from build123d import *

# Parameters (mm, degrees)
SKETCH1_W               = 20
SKETCH1_H               = 20
SKETCH1_R               = 1.5
SKETCH1_R_2             = 8
BOSS_EXTRUDE1_DEPTH     = 2.5
SKETCH2_R               = 3.175
BOSS_EXTRUDE2_DEPTH     = 20
CUT_EXTRUDE2_DEPTH      = 27.119915773
CUT_EXTRUDE2_DEPTH_BACK = 27.119915773
SKETCH1_3_R             = 1.5


with BuildPart() as part:
    # Sketch1 → Boss-Extrude1 (new body)
    # profile 1 of 18: a face of its own
    with BuildSketch(Plane(origin=(0, 0, 0), x_dir=(1, 0, 0), z_dir=(0, 1, 0))):
        with Locations((0, -10)):
            Rectangle(SKETCH1_W, SKETCH1_H)
        with Locations((0, -2)):
            Circle(SKETCH1_R, mode=Mode.SUBTRACT)
        with Locations((0, -10)):
            Circle(SKETCH1_R_2, mode=Mode.SUBTRACT)
        with Locations((8, -10)):
            Circle(SKETCH1_R, mode=Mode.SUBTRACT)
        with Locations((0, -18)):
            Circle(SKETCH1_R, mode=Mode.SUBTRACT)
        with Locations((-8, -10)):
            Circle(SKETCH1_R, mode=Mode.SUBTRACT)
    # profile 2 of 18: a face of its own
    with BuildSketch(Plane(origin=(0, 0, 0), x_dir=(1, 0, 0), z_dir=(0, 1, 0))):
        with Locations((8, -10)):
            Circle(SKETCH1_R)
    # profile 3 of 18: a face of its own
    with BuildSketch(Plane(origin=(0, 0, 0), x_dir=(1, 0, 0), z_dir=(0, 1, 0))):
        with Locations((0, -18)):
            Circle(SKETCH1_R)
    # profile 4 of 18: a face of its own
    with BuildSketch(Plane(origin=(0, 0, 0), x_dir=(1, 0, 0), z_dir=(0, 1, 0))):
        with Locations((-8, -10)):
            Circle(SKETCH1_R)
    # profile 5 of 18: a face of its own
    with BuildSketch(Plane(origin=(0, 0, 0), x_dir=(1, 0, 0), z_dir=(0, 1, 0))):
        with Locations((0, -10)):
            Circle(SKETCH1_R_2)
    # profile 6 of 18: a face of its own
    with BuildSketch(Plane(origin=(0, 0, 0), x_dir=(1, 0, 0), z_dir=(0, 1, 0))):
        with Locations((0, -2)):
            Circle(SKETCH1_R)
    # profile 7 of 18: a face of its own
    with BuildSketch(Plane(origin=(0, 0, 0), x_dir=(1, 0, 0), z_dir=(0, 1, 0))):
        with Locations((0, -10)):
            Circle(SKETCH1_R_2)
    # profile 8 of 18: a face of its own
    with BuildSketch(Plane(origin=(0, 0, 0), x_dir=(1, 0, 0), z_dir=(0, 1, 0))):
        with Locations((8, -10)):
            Circle(SKETCH1_R)
    # profile 9 of 18: a face of its own
    with BuildSketch(Plane(origin=(0, 0, 0), x_dir=(1, 0, 0), z_dir=(0, 1, 0))):
        with Locations((0, -10)):
            Circle(SKETCH1_R_2)
    # profile 10 of 18: a face of its own
    with BuildSketch(Plane(origin=(0, 0, 0), x_dir=(1, 0, 0), z_dir=(0, 1, 0))):
        with Locations((0, -18)):
            Circle(SKETCH1_R)
    # profile 11 of 18: a face of its own
    with BuildSketch(Plane(origin=(0, 0, 0), x_dir=(1, 0, 0), z_dir=(0, 1, 0))):
        with Locations((0, -10)):
            Circle(SKETCH1_R_2)
    # profile 12 of 18: a face of its own
    with BuildSketch(Plane(origin=(0, 0, 0), x_dir=(1, 0, 0), z_dir=(0, 1, 0))):
        with Locations((0, -18)):
            Circle(SKETCH1_R)
    # profile 13 of 18: a face of its own
    with BuildSketch(Plane(origin=(0, 0, 0), x_dir=(1, 0, 0), z_dir=(0, 1, 0))):
        with Locations((0, -10)):
            Circle(SKETCH1_R_2)
    # profile 14 of 18: a face of its own
    with BuildSketch(Plane(origin=(0, 0, 0), x_dir=(1, 0, 0), z_dir=(0, 1, 0))):
        with Locations((-8, -10)):
            Circle(SKETCH1_R)
    # profile 15 of 18: a face of its own
    with BuildSketch(Plane(origin=(0, 0, 0), x_dir=(1, 0, 0), z_dir=(0, 1, 0))):
        with Locations((0, -10)):
            Circle(SKETCH1_R_2)
    # profile 16 of 18: a face of its own
    with BuildSketch(Plane(origin=(0, 0, 0), x_dir=(1, 0, 0), z_dir=(0, 1, 0))):
        with Locations((-8, -10)):
            Circle(SKETCH1_R)
    # profile 17 of 18: a face of its own
    with BuildSketch(Plane(origin=(0, 0, 0), x_dir=(1, 0, 0), z_dir=(0, 1, 0))):
        with Locations((0, -10)):
            Circle(SKETCH1_R_2)
    # profile 18 of 18: a face of its own
    with BuildSketch(Plane(origin=(0, 0, 0), x_dir=(1, 0, 0), z_dir=(0, 1, 0))):
        with Locations((8, -10)):
            Circle(SKETCH1_R)
    extrude(amount=BOSS_EXTRUDE1_DEPTH)

    # Sketch2 → Boss-Extrude2 (add)
    with BuildSketch(Plane.ZY.offset(10)):
        with BuildLine():
            Line((0, 0), (20, 0))
            Line((20, 0), (20, -3.5))
            ThreePointArc((20, -3.5), (10, -13.5), (0, -3.5))
            Line((0, -3.5), (0, 0))
        make_face()
        with Locations((10, -3.5)):
            Circle(SKETCH2_R, mode=Mode.SUBTRACT)
    extrude(amount=-BOSS_EXTRUDE2_DEPTH)

    # Sketch1<3> → Cut-Extrude2 (cut, two sides: drawn at the far end of the back side and taken through both)
    with BuildSketch(Plane(origin=(0, 0, 0), x_dir=(1, 0, 0), z_dir=(0, 1, 0)).offset(-CUT_EXTRUDE2_DEPTH_BACK)):
        with Locations(Location((8, -10, 0), (0, 0, 270))):
            Circle(SKETCH1_3_R)
        with Locations(Location((0, -18, 0), (0, 0, 270))):
            Circle(SKETCH1_3_R)
        with Locations(Location((-8, -10, 0), (0, 0, 270))):
            Circle(SKETCH1_3_R)
        with Locations(Location((0, -2, 0), (0, 0, 270))):
            Circle(SKETCH1_3_R)
    extrude(amount=CUT_EXTRUDE2_DEPTH + CUT_EXTRUDE2_DEPTH_BACK, mode=Mode.SUBTRACT)


solid = part.part
Design review of the part built by this model. Coordinates are the model's own, in mm. Coordinates: 2 decimals unless noted, no trailing zeros. Loops run counter-clockwise (first coordinate to the right, second up) from the corner with the lowest first, then second, coordinate; pieces in that order, holes last.
Item 1: Draft analysis for pull direction Z (two halves, no side actions). For faces 1 (the flat face through (10, -7, 10)), 2 (the cylindrical face through (6.536, 0.877, 9.675)), 3 (the flat face through (0, 0, 20)), state which applies: pulls with the +Z half, pulls with the -Z half, needs draft (parallel to the pull), parting line crosses it, or undercut.
Completed:
face 1: needs draft
face 2: undercut
face 3: pulls with the +Z half
Item 2: Add section A-A (z = 2). Write out the cut boundary in (x, y), and give its area (3 significant figures).
Completed:
outline: (-10, -9.5) - (-1.5, -9.5) - (-1.5, 2.5) - (-10, 2.5) - close; (1.5, -9.5) - (10, -9.5) - (10, 2.5) - (1.5, 2.5) - close
area: 204 mm2
Item 3: Clearance check with flat-ended pins moving along their axes: pin 1 (3.5 mm diameter, centred on x = 0, z = 18, fed in from -Y); pin 2 (5 mm diameter, centred on x = 0, z = 2, fed in from -Y). State where each tip first meets the part, or that it passes through.
Completed:
pin 1: stops at y = -11.31
pin 2: stops at y = -11.85
Item 4: Add section B-B (z = 10). Write out the cut boundary in (x, y) (3 decimals).
Completed:
outline: (-10, -13.5) - (-9.5, -13.5) - (-9.5, -6.675) - (-10, -6.675) - close; (-10, -0.325) - (-9.5, -0.325) - (-9.5, 2.5) - (-10, 2.5) - close; (-6.5, -13.5) - (6.5, -13.5) - (6.5, -6.675) - (-6.5, -6.675) - close; (-6.5, -0.325) - (6.5, -0.325) - (6.5, 2.5) - (-6.5, 2.5) - close; (9.5, -13.5) - (10, -13.5) - (10, -6.675) - (9.5, -6.675) - close; (9.5, -0.325) - (10, -0.325) - (10, 2.5) - (9.5, 2.5) - close
Item 5: Add section D-D (x = -1). Write out the cut boundary in (y, z) (3 decimals), and give its area (3 significant figures).
Completed:
outline: (-10.755, 3.118) - (2.5, 3.118) - (2.5, 16.882) - (-10.755, 16.882) arc R10 ccw to start; (-7.606, 0.882) arc R10 ccw to (-3.5, 0) - (2.5, 0) - (2.5, 0.882) - close; (-7.606, 19.118) - (2.5, 19.118) - (2.5, 20) - (-3.5, 20) arc R10 ccw to start; hole circle Ø6.35 at (-3.5, 10)
area: 192 mm2
Item 6: Wall thickness on L1, parallel to X at y = -10.5, z = 10; L2, parallel to X at y = 0.5, z = 18; L3, parallel to X at y = -7, z = 10.5: over which ranges is each line inside the solid? List them lowest first.
Completed:
L1: x = -10 to -9.5, -6.5 to 6.5, 9.5 to 10
L2: x = -10 to -1.5, 1.5 to 10
L3: x = -10 to -9.41, -6.59 to 6.59, 9.41 to 10
Item 7: Add section C-C (y = 1.25). Write out the cut boundary in (x, z), and give its area (3 significant figures).
Completed:
outline: (-10, 0) - (10, 0) - (10, 20) - (-10, 20) - close; hole circle Ø3 at (-8, 10); hole circle Ø3 at (0, 2); hole circle Ø3 at (0, 18); hole circle Ø3 at (8, 10)
area: 372 mm2
